Verification items for this drawing (mm, ordinates from the low corner). A direction names the side the tool comes from. Coordinates: 2 decimals unless noted, no trailing zeros. Order: outer loops, then holes, each group sorted by start corner. A loop starts at its lowest first (then second) coordinate and runs counter-clockwise, first axis right, second up. Notation, with made-up numbers: (-27.5, -24.5) -> (4.5, -24.5) arc R25 ccw to (4.5, 3.5) -> close; hole circle Ø6 at (-33, 1). An arc over 180 degrees is marked (long way). Put each result on its own line as item: value. Start each with the question number.
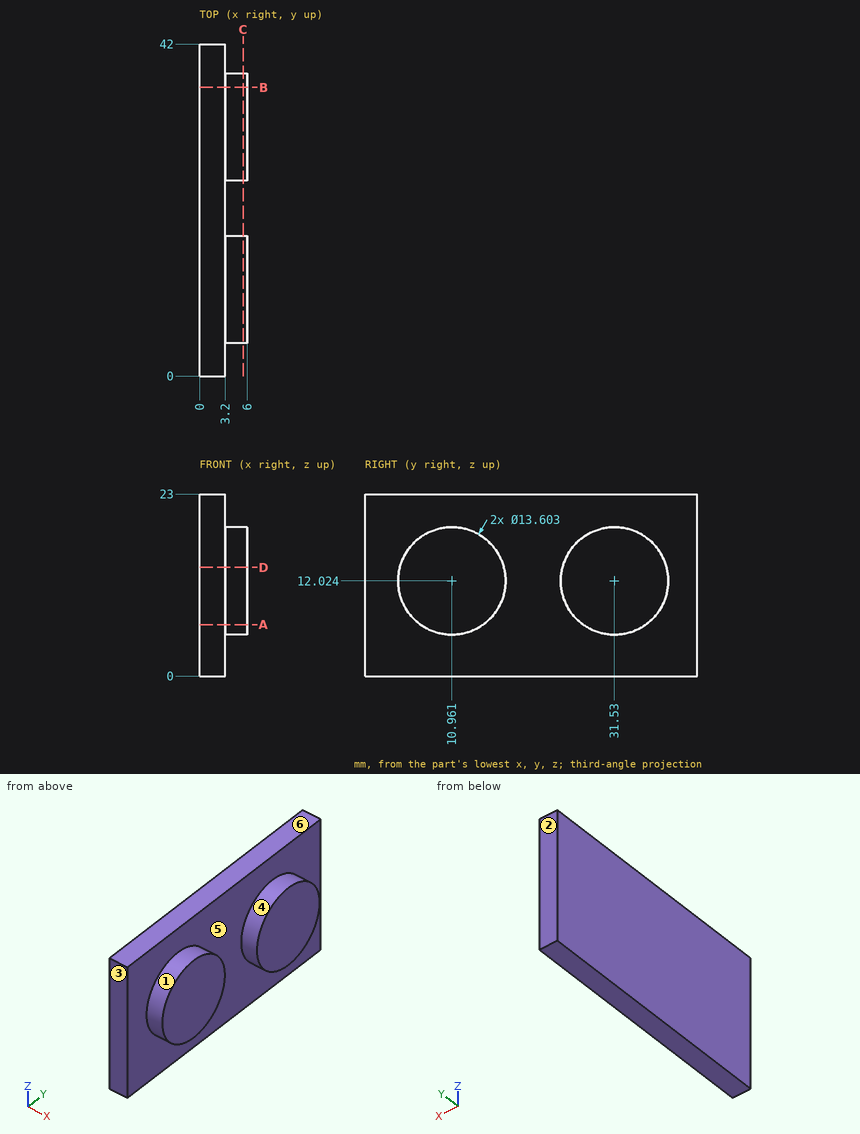
1) Sectioned sample at C-C (x = 5.5). Record the boundary of the cut face in (y, z).
2) Sectioned sample at A-A (z = 6.5). Record the boundary of the cut face in (x, y).
3) Access from +Z, -Z, +X, -X, +Y, -Y to the whole of each face (thin tool, end or side, straight path). Record for the marked faces 1 and 2.
4) Scan lines: line 1 along X through (y, z) = (21, 14.5); line 2 along Y through (x, z) = (3.7, 7.75); line 3 along Y through (x, z) = (3.9, 18.25) (1 decimal). Record each from-to range of solid material in increasing order. Write a range as [from, to].
5) Sectioned sample at B-B (y = 36.5). Record the boundary of the cut face in (x, z).
6) Mould release check, pull along Y, two halves, no side actions. Record for the marked faces 3, 4, 5 and 6: +Y half, -Y half, draft (parallel to the pull), parting line (faces both ways), or undercut.
7) Sectioned sample at D-D (z = 13.75). Record the boundary of the cut face in (x, y), plus the area to 3 significant figures.
Entries:
1. outline: circle Ø13.6 at (10.96, 12.02); circle Ø13.6 at (31.53, 12.02)
2. outline: (0, 0) -> (3.2, 0) -> (3.2, 6.99) -> (6, 6.99) -> (6, 14.93) -> (3.2, 14.93) -> (3.2, 27.56) -> (6, 27.56) -> (6, 35.5) -> (3.2, 35.5) -> (3.2, 42) -> (0, 42) -> close
3. face 1: +X
3. face 2: +Z, -Z, +X, -X, +Y
4. line 1: x = [0, 3.2]
4. line 2: y = [5.67, 16.25], [26.24, 36.82]
4. line 3: y = [8.2, 13.7], [28.8, 34.3]
5. outline: (0, 0) -> (3.2, 0) -> (3.2, 7.38) -> (6, 7.38) -> (6, 16.67) -> (3.2, 16.67) -> (3.2, 23) -> (0, 23) -> close
6. face 3: -Y half
6. face 4: undercut
6. face 5: undercut
6. face 6: draft
7. outline: (0, 0) -> (3.2, 0) -> (3.2, 4.38) -> (6, 4.38) -> (6, 17.54) -> (3.2, 17.54) -> (3.2, 24.95) -> (6, 24.95) -> (6, 38.11) -> (3.2, 38.11) -> (3.2, 42) -> (0, 42) -> close
7. area: 208 mm2
